Verification items for the finished model (mm, model axes). A direction names the side the tool comes from. Coordinates: 2 decimals unless noted, no trailing zeros. Write each loop counter-clockwise with the first axis right and the second up, starting at its lowest first coordinate (ties: lowest second). Pieces come first, ordered by that corner, then holes. Notation, with made-up numbers: (-2, -27.5) -> (52, -27.5) arc R27 cw to (52, -0.5) -> close; hole circle Ø6 at (8, 6.5). An arc over 180 degrees is marked (long way). Answer in a Markdown table with one row per item.
```python
from build123d import *

# Parameters (mm, degrees)
PAD_DEPTH       = 80
SKETCH001_R     = 1.6
POCKET_DEPTH    = 13.501
SKETCH002_R     = 3
POCKET001_DEPTH = 5
SKETCH003_R     = 10.65
POCKET002_DEPTH = 30.4
SKETCH004_R     = 10.65
POCKET003_DEPTH = 30.4
FILLET_R        = 5


with BuildPart() as part:
    # Sketch → Pad (new body)
    with BuildSketch(Plane.XZ):
        with BuildLine():
            Line((20, 0), (20, -13.5))
            Line((20, -13.5), (-20, -13.5))
            Line((-20, -13.5), (-20, 0))
            Line((-20, 0), (-7, 0))
            ThreePointArc((-7, 0), (0, -7), (7, 0))
            Line((7, 0), (20, 0))
        make_face()
    extrude(amount=PAD_DEPTH)

    # Sketch001 → Pocket (cut, through all)
    with BuildSketch(Plane.XY):
        with Locations((-15, -5)):
            Circle(SKETCH001_R)
        with Locations((-15, -40)):
            Circle(SKETCH001_R)
        with Locations((-15, -75)):
            Circle(SKETCH001_R)
        with Locations((15, -5)):
            Circle(SKETCH001_R)
        with Locations((15, -40)):
            Circle(SKETCH001_R)
        with Locations((15, -75)):
            Circle(SKETCH001_R)
    extrude(amount=-POCKET_DEPTH, mode=Mode.SUBTRACT)

    # Sketch002 (on DatumPlane) → Pocket001 (cut)
    with BuildSketch(Plane.XY.offset(-13.5)):
        with Locations((-15, -5)):
            Circle(SKETCH002_R)
        with Locations((-15, -40)):
            Circle(SKETCH002_R)
        with Locations((-15, -75)):
            Circle(SKETCH002_R)
        with Locations((15, -5)):
            Circle(SKETCH002_R)
        with Locations((15, -40)):
            Circle(SKETCH002_R)
        with Locations((15, -75)):
            Circle(SKETCH002_R)
    extrude(amount=POCKET001_DEPTH, mode=Mode.SUBTRACT)

    # Sketch003 (on DatumPlane) → Pocket002 (cut)
    with BuildSketch(Plane.XZ.offset(5)):
        Circle(SKETCH003_R)
    extrude(amount=POCKET002_DEPTH, mode=Mode.SUBTRACT)

    # Sketch004 (on DatumPlane) → Pocket003 (cut)
    with BuildSketch(Plane.XZ.offset(75)):
        Circle(SKETCH004_R)
    extrude(amount=-POCKET003_DEPTH, mode=Mode.SUBTRACT)

    # Fillet
    fillet_edges = [part.edges().sort_by_distance(p)[0] for p in [
        (-20, -80, -6.75),
    ]]
    fillet(fillet_edges, radius=FILLET_R)


solid = part.part
```
1. Section check B-B, the plane z = -6. State how many separate pieces and enclosed holes the cut face has, plus the area to 3 significant figures.
Geometry says:
| item | result |
|---|---|
| separate pieces | 2 |
| enclosed holes | 6 |
| area | 1,940 mm^2 |
2. Section check A-A, the plane x = 15. Record the boundary of the cut face in (y, z), plus the area to 3 significant figures.
Geometry says:
| item | result |
|---|---|
| outline | (-80, -13.5) -> (-78, -13.5) -> (-78, -8.5) -> (-76.6, -8.5) -> (-76.6, 0) -> (-80, 0) -> close; (-73.4, -8.5) -> (-72, -8.5) -> (-72, -13.5) -> (-43, -13.5) -> (-43, -8.5) -> (-41.6, -8.5) -> (-41.6, 0) -> (-73.4, 0) -> close; (-38.4, -8.5) -> (-37, -8.5) -> (-37, -13.5) -> (-8, -13.5) -> (-8, -8.5) -> (-6.6, -8.5) -> (-6.6, 0) -> (-38.4, 0) -> close; (-3.4, -8.5) -> (-2, -8.5) -> (-2, -13.5) -> (0, -13.5) -> (0, 0) -> (-3.4, 0) -> close |
| area | 908 mm^2 |
3. Section check D-D, the plane x = 0. Record the boundary of the cut face in (y, z), plus the area to 3 significant figures.
Geometry says:
| item | result |
|---|---|
| outline | (-80, -13.5) -> (0, -13.5) -> (0, -7) -> (-5, -7) -> (-5, -10.65) -> (-35.4, -10.65) -> (-35.4, -7) -> (-44.6, -7) -> (-44.6, -10.65) -> (-75, -10.65) -> (-75, -7) -> (-80, -7) -> close |
| area | 298 mm^2 |
4. Mould release check, pull along Y, two halves, no side actions. Record for faces 1 (the cylindrical face through (0, -40, -7)), 2 (the flat face through (16.3, -41.3, -8.5)), 3 (the cylindrical face through (-18, -79, -7)): released by +Y, released by -Y, zero draft, split by the parting line, or undercut.
Geometry says:
| item | result |
|---|---|
| face 1 | zero draft |
| face 2 | undercut |
| face 3 | released by -Y |
5. Section check C-C, the plane y = -40. Record the boundary of the cut face in (x, z).
Geometry says:
| item | result |
|---|---|
| outline | (-20, -13.5) -> (-18, -13.5) -> (-18, -8.5) -> (-16.6, -8.5) -> (-16.6, 0) -> (-20, 0) -> close; (-13.4, -8.5) -> (-12, -8.5) -> (-12, -13.5) -> (12, -13.5) -> (12, -8.5) -> (13.4, -8.5) -> (13.4, 0) -> (7, 0) arc R7 cw to (-7, 0) -> (-13.4, 0) -> close; (16.6, -8.5) -> (18, -8.5) -> (18, -13.5) -> (20, -13.5) -> (20, 0) -> (16.6, 0) -> close |
6. Tool access check on faces 4 (the flat face through (0, -44.6, -8)), 5 (the cylindrical face through (-15.65, -77.93, -11.04)), 6 (the flat face through (0, 0, -8)). Record the directions out of +Z, -Z, +X, -X, +Y, -Y that give a thin tool (end or side, any length) a straight path to the whole face; none if there is none.
Geometry says:
| item | result |
|---|---|
| face 4 | +Z |
| face 5 | -Z |
| face 6 | +Z, -Z, +X, -X, +Y |
7. Depth check by flat-ended pin: P1, Ø6.5, axis at x = 14, y = -40.5, coming from the -Z side; P2, Ø3, axis at x = -14.5, y = -74.5, coming from the -Z side; P3, Ø8, axis at x = 1.5, y = -51, coming from the +Z side. Enter the tip coordinate at first touch or a pass-through.
Geometry says:
| item | result |
|---|---|
| P1 | z = -13.5 |
| P2 | z = -8.5 |
| P3 | z = -9.12 |
8. Thickness scan on line 1 (Y direction, x = 1.5, z = -8.5); line 2 (Y direction, x = -15, z = -4.5); line 3 (Y direction, x = -15, z = -10.4). Record the ranges inside material, lowest first. Write a range as from..to.
Geometry says:
| item | result |
|---|---|
| line 1 | -80..-75, -44.6..-35.4, -5..0 |
| line 2 | -80..-76.6, -73.4..-41.6, -38.4..-6.6, -3.4..0 |
| line 3 | -80..-78, -72..-43, -37..-8, -2..0 |
